Design review of the part shown in the three views and the two pictorial views. Dimensions are in mm from the part's minimum x, y and z. A direction names the side the tool comes from. Round coordinates to 2 decimals unless told otherwise and drop trailing zeros. Write each loop counter-clockwise with the first axis right and the second up, starting at its lowest first coordinate (ties: lowest second). Pieces come first, ordered by that corner, then holes. Notation, with made-up numbers: (19.5, 67) - (71.5, 67) arc R32 ccw to (71.5, 103) - close; hole circle Ø1 at (-16, 81). An arc over 180 degrees is marked (long way). Use one line per item in the form item = value.
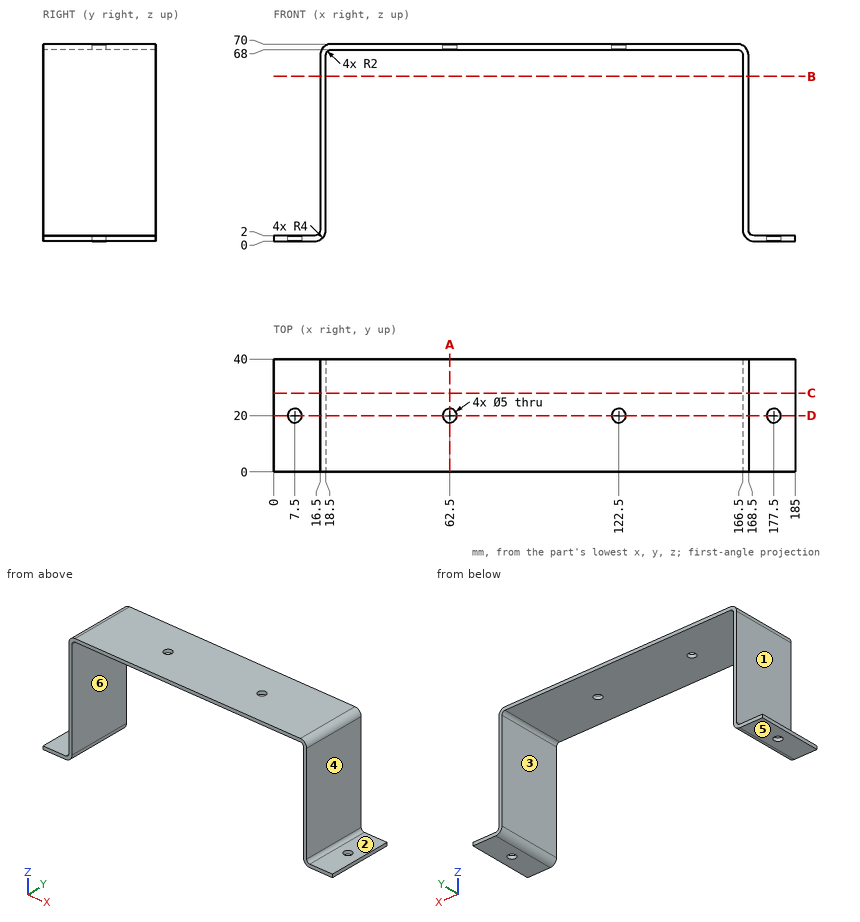
Q1. We need section A-A on x = 62.5. Write out the cut boundary in (y, z), then the cut area to 3 significant figures.
Calculated:
outline = (0, 68) - (17.5, 68) - (17.5, 70) - (0, 70) - close; (22.5, 68) - (40, 68) - (40, 70) - (22.5, 70) - close
area = 70.0 mm2
Q2. Machinability: for the marked faces 4, 5 and 6, which of the approach directions +Z, -Z, +X, -X, +Y, -Y give a long, thin tool a straight path to every point of the face, cutting with its end or side? Answer none if there is none.
Calculated:
face_4 = +Z, +X, +Y, -Y
face_5 = -Z, +X, -X, +Y, -Y
face_6 = -Z, +Y, -Y
Q3. We need section D-D on y = 20. State how many separate pieces and enclosed holes the cut face has, then the cut area to 3 significant figures.
Calculated:
separate_pieces = 5
enclosed_holes = 0
area = 592 mm2
Q4. We need section C-C on y = 28. Write out the cut boundary in (x, z), then the cut area to 3 significant figures.
Calculated:
outline = (0, 0) - (14.5, 0) arc R4 ccw to (18.5, 4) - (18.5, 66) arc R2 cw to (20.5, 68) - (164.5, 68) arc R2 cw to (166.5, 66) - (166.5, 4) arc R4 ccw to (170.5, 0) - (185, 0) - (185, 2) - (170.5, 2) arc R2 cw to (168.5, 4) - (168.5, 66) arc R4 ccw to (164.5, 70) - (20.5, 70) arc R4 ccw to (16.5, 66) - (16.5, 4) arc R2 cw to (14.5, 2) - (0, 2) - close
area = 632 mm2
Q5. We need section B-B on z = 58.5. Write out the cut boundary in (x, y), then the cut area to 3 significant figures.
Calculated:
outline = (16.5, 0) - (18.5, 0) - (18.5, 40) - (16.5, 40) - close; (166.5, 0) - (168.5, 0) - (168.5, 40) - (166.5, 40) - close
area = 160 mm2
Q6. For P1, Ø4, axis at y = 15.5, z = 26.5, coming from the -X side; P2, Ø3, axis at x = 51.5, y = 6, coming from the -Z side; P3, Ø11.5, axis at x = 9.5, y = 13, coming from the +Z side, all flat-tipped, find the tip position at first contact; note any pin that passes through.
Calculated:
P1 = 16.5
P2 = 68
P3 = 2.15
Q7. Draft analysis for pull direction X (two halves, no side actions). For the marked faces 1, 2 and 3, state which applies: released by +X, released by -X, zero draft, split by the parting line, or undercut.
Calculated:
face_1 = released by -X
face_2 = zero draft
face_3 = undercut
Q8. To check wall thickness, follow line 1 along Y through (x, z) = (177.5, 1.4); line 2 along X through (y, z) = (17.5, 39); line 3 along X through (y, z) = (36, 3). State the ranges of each line that lie inside material, in increasing order. Write a range as from..to.
Calculated:
line_1 = 0..17.5, 22.5..40
line_2 = 16.5..18.5, 166.5..168.5
line_3 = 16.23..18.37, 166.63..168.77
